from build123d import *

# Parameters (mm, degrees)
SKETCH_1_R          = 2
EXTRUDE_1_DEPTH     = 18
CUT_EXTRUDE_START   = -7
SKETCH_2_R          = 2
SKETCH_2_R_2        = 1.8
CUT_EXTRUDE_1_DEPTH = 0.5


with BuildPart() as part:
    # 草图1 → 凸台-拉伸1 (new body)
    with BuildSketch(Plane(origin=(0, 0, 0), x_dir=(0, 0, -1), z_dir=(1, 0, 0))):
        Circle(SKETCH_1_R)
    extrude(amount=EXTRUDE_1_DEPTH)

    # 草图2 → 切除-拉伸1 (cut)
    with BuildSketch(Plane(origin=(18, 0, 0), x_dir=(0, 0, -1), z_dir=(1, 0, 0)).offset(CUT_EXTRUDE_START)):
        Circle(SKETCH_2_R)
        Circle(SKETCH_2_R_2, mode=Mode.SUBTRACT)
    cut_extrude_1 = extrude(amount=CUT_EXTRUDE_1_DEPTH, mode=Mode.SUBTRACT)

    # 镜向1: 切除-拉伸1 across plane
    add(cut_extrude_1.mirror(Plane(origin=(9, 0, 0), x_dir=(0, 0, 1), z_dir=(1, 0, 0))), mode=Mode.SUBTRACT)


solid = part.part
The model under review builds one solid part; all positions refer to its coordinate system, in mm. A direction names the side the tool comes from. Round coordinates to 2 decimals unless told otherwise and drop trailing zeros. Loops run counter-clockwise (first coordinate to the right, second up) from the corner with the lowest first, then second, coordinate; pieces in that order, holes last. Notation, with made-up numbers: (31, 6) - (39, 6) arc R33 ccw to (39, 35) - close; hole circle Ø9 at (81.5, -18). An arc over 180 degrees is marked (long way). Use CSV: the item, a comma, the result in double quotes.
(1) For line 1 (X direction, y = -1.6, z = 1.15); line 2 (Y direction, x = 8.5, z = -1.3); line 3 (Z direction, x = 13.75, y = -0.2), list the stretches that pass through material, from the lowest coordinate up.
Working result:
line 1,"x = 0 to 6.5, 7 to 11, 11.5 to 18"
line 2,"y = -1.52 to 1.52"
line 3,"z = -1.99 to 1.99"
(2) Take a section at A-A, the plane x = 4.75. Give the boundary of the cut face in (y, z), plus the area to 3 significant figures.
Working result:
outline,"circle Ø4 at (0, 0)"
area,"12.6 mm^2"
(3) Take a section at B-B, the plane y = -0.35. Give the boundary of the cut face in (x, z).
Working result:
outline,"(0, -1.97) - (6.5, -1.97) - (6.5, -1.77) - (7, -1.77) - (7, -1.97) - (11, -1.97) - (11, -1.77) - (11.5, -1.77) - (11.5, -1.97) - (18, -1.97) - (18, 1.97) - (11.5, 1.97) - (11.5, 1.77) - (11, 1.77) - (11, 1.97) - (7, 1.97) - (7, 1.77) - (6.5, 1.77) - (6.5, 1.97) - (0, 1.97) - close"
(4) Machinability: for faces 4 (the cylindrical face through (11.246, 0.541, -1.717)), 5 (the flat face through (18, 0, 0)), which of the approach directions +Z, -Z, +X, -X, +Y, -Y give a long, thin tool a straight path to every point of the face, cutting with its end or side? Answer none if there is none.
Working result:
face 4,"none"
face 5,"+Z, -Z, +X, +Y, -Y"
(5) The part is to be moulded in two halves that separate along X. For faces 1 (the cylindrical face through (15, -2, 0)), 2 (the flat face through (0, 0, 0)), 3 (the cylindrical face through (6.754, 0.541, -1.717)), say which applies: pulls with the +X half, pulls with the -X half, needs draft (parallel to the pull), parting line crosses it, or undercut.
Working result:
face 1,"needs draft"
face 2,"pulls with the -X half"
face 3,"undercut"
